Geometry: final body of the model. Coordinates: model frame, mm. A direction names the side the tool comes from. Coordinates: 2 decimals unless noted, no trailing zeros. Loops run counter-clockwise (first coordinate to the right, second up) from the corner with the lowest first, then second, coordinate; pieces in that order, holes last. Notation, with made-up numbers: (50.25, -30) -> (107.25, -30) arc R24 ccw to (107.25, -6) -> close; hole circle Ø5 at (83, -18.5). An arc over 180 degrees is marked (long way). One line per item, written item: value. Start each with the question number.
from build123d import *

# Parameters (mm, degrees)
F0_R     = 9
F1_DEPTH = 105
F2_SIZE  = 1
F5_DEPTH = 25


with BuildPart() as f1:
    # F0 (on Front) → F1 (new body)
    with BuildSketch(Plane.XZ):
        Circle(F0_R)
    extrude(amount=F1_DEPTH)

    # F2
    f2_edges = [f1.edges().sort_by_distance(p)[0] for p in [
        (9, -52.5, 0),
        (-9, 0, 0),
        (-9, -105, 0),
    ]]
    chamfer(f2_edges, length=F2_SIZE)

    # F4 (on offset) → F5 (cut)
    with BuildSketch(Plane.XY.offset(6)):
        with BuildLine():
            Line((3, -29), (3, -11))
            ThreePointArc((3, -11), (0, -8), (-3, -11))
            Line((-3, -11), (-3, -29))
            ThreePointArc((-3, -29), (0, -32), (3, -29))
        make_face()
    extrude(amount=F5_DEPTH, mode=Mode.SUBTRACT)


solid = f1.part
1. Section B-B on y = -68. Return the cut outline in (x, z), plus the area to 3 significant figures.
2. Pin query (flat end, axial travel): pin 1 Ø1 at (y, z) = (-29, 7) entering from +X; pin 2 Ø4 at (y, z) = (-25, -6.5) entering from +X; pin 3 Ø0.7 at (y, z) = (-20, 7.5) entering from +X. Return the tip coordinate at first contact, or that it passes through.
3. Section A-A on y = -14. Return the cut outline in (x, z).
4. Draft query along X for faces 1 (the face through (0, -32, 7)), 2 (the face through (0, -105, 0)), 3 (the face through (-1.951, -51.779, -8.786)). Return one class per face: released by +X, released by -X, zero draft, split by the parting line, or undercut.
5. Set-up query: faces 4 (the face through (0, -8, 7)), 5 (the face through (0, 0, 0)). Return all of +Z, -Z, +X, -X, +Y, -Y with unobstructed straight access to the full face (end or side cutting, diameter ignored); none if empty.
6. Line query: L1, parallel to X at y = -73.5, z = 0.5; L2, parallel to Y at x = 0, z = 7; L3, parallel to X at y = -16.5, z = 8. Output: solid intervals per line, ascending. Write a range as [from, to].
Checks:
1. outline: circle Ø18 at (0, 0)
1. area: 254 mm²
2. pin 1: x = 6.22
2. pin 2: x = 7.79
2. pin 3: x = 5.47
3. outline: (-3, 6) -> (-3, 8.49) arc R9 ccw (long way) to (3, 8.49) -> (3, 6) -> close
4. face 1: undercut
4. face 2: zero draft
4. face 3: split by the parting line
5. face 4: +Z
5. face 5: +Z, -Z, +X, -X, +Y
6. L1: [-8.99, 8.99]
6. L2: [-105, -32], [-8, 0]
6. L3: [-4.12, -3], [3, 4.12]
